from build123d import *

# Parameters (mm, degrees)
SKETCH1_R           = 14
BOSS_EXTRUDE1_DEPTH = 5
BOSS_EXTRUDE3_DEPTH = 20
SKETCH3_R           = 8.5
CUT_EXTRUDE1_DEPTH  = 26
SKETCH5_W           = 4
SKETCH5_H           = 11.5
CUT_EXTRUDE3_DEPTH  = 26
SKETCH6_R           = 1.5
CUT_EXTRUDE4_DEPTH  = 6
CIRPATTERN1_COUNT   = 3
FILLET1_R           = 1.5


with BuildPart() as part:
    # Sketch1 → Boss-Extrude1 (new body)
    with BuildSketch(Plane.XY):
        Circle(SKETCH1_R)
    extrude(amount=BOSS_EXTRUDE1_DEPTH)

    # Sketch2 → Boss-Extrude3 (add)
    with BuildSketch(Plane.XY.offset(5)):
        with BuildLine():
            Line((2.5, -9.16515139), (2.5, -12.16515139))
            Line((2.5, -12.16515139), (-2.5, -12.16515139))
            Line((-2.5, -12.16515139), (-2.5, -9.16515139))
            ThreePointArc((-2.5, -9.16515139), (0, 9.5), (2.5, -9.16515139))
        make_face()
    extrude(amount=BOSS_EXTRUDE3_DEPTH)

    # Sketch3 → Cut-Extrude1 (cut, through all)
    with BuildSketch(Plane.XY.offset(25)):
        Circle(SKETCH3_R)
    extrude(amount=-CUT_EXTRUDE1_DEPTH, mode=Mode.SUBTRACT)

    # Sketch5 → Cut-Extrude3 (cut, through all)
    with BuildSketch(Plane.XY.offset(25)):
        with Locations((0, -5.75)):
            Rectangle(SKETCH5_W, SKETCH5_H)
    extrude(amount=-CUT_EXTRUDE3_DEPTH, mode=Mode.SUBTRACT)

    # Sketch6 → Cut-Extrude4 (cut, through all)
    with BuildSketch(Plane.XY.offset(5)):
        with Locations((0, 11.75)):
            Circle(SKETCH6_R)
    cut_extrude4 = extrude(amount=-CUT_EXTRUDE4_DEPTH, mode=Mode.SUBTRACT)

    # CirPattern1: Cut-Extrude4 ×3 about axis
    cirpattern1_axis = Axis((0, 0, 0), (0, 0, 1))
    for i in range(1, CIRPATTERN1_COUNT):
        add(cut_extrude4.rotate(cirpattern1_axis, i * 360 / CIRPATTERN1_COUNT), mode=Mode.SUBTRACT)

    # Fillet1
    fillet1_edges = [part.edges().sort_by_distance(p)[0] for p in [
        (2, -8.261355821, 12.5),
        (-2, -8.261355821, 12.5),
    ]]
    fillet(fillet1_edges, radius=FILLET1_R)


solid = part.part
The listing builds one solid part. Answer for the finished solid, in the listing's coordinates (mm). A direction names the side the tool comes from. Give positions to 0.01 mm unless a question says otherwise; leave off trailing zeros. Loops run counter-clockwise (first coordinate to the right, second up) from the corner with the lowest first, then second, coordinate; pieces in that order, holes last.
Item 1: Each of these flat-tipped pins is pushed along its axis until it touches: pin 1 Ø1.5 at (x, z) = (-7, 14.5) entering from -Y; pin 2 Ø4.5 at (x, z) = (-0.5, 10.5) entering from +Y; pin 3 Ø12 at (y, z) = (-6, 21.5) entering from -X; pin 4 Ø5 at (y, z) = (0.5, 3.5) entering from +X. Where does it stop, or does it pass through?
Derived:
pin 1: stops at y = -7.15
pin 2: stops at y = 9.5
pin 3: stops at x = -9.5
pin 4: stops at x = 14
Item 2: Find the intervals of material crossed by line 1 along X through (y, z) = (-10.5, 6); line 2 along X through (y, z) = (-6.25, 3); line 3 along X through (y, z) = (0, 13), in increasing order.
Derived:
line 1: x = -2.5 to -2, 2 to 2.5
line 2: x = -12.53 to -11.63, -8.72 to -5.76, 5.76 to 8.72, 11.63 to 12.53
line 3: x = -9.5 to -8.5, 8.5 to 9.5
Item 3: Determine the mould class of faces 1 (the cylindrical face through (-0.382, 9.492, 14.86)), 2 (the flat face through (-2, -10, 13)), 3 (the flat face through (4, -8, 25)) for opening direction Y: +Y half, -Y half, draft (parallel to the pull), parting line (faces both ways), or undercut.
Derived:
face 1: parting line
face 2: undercut
face 3: draft
Item 4: A cutting plane is placed at B-B (y = 0). Give the vertices of the cut face in (x, z), then the cut area to 3 significant figures.
Derived:
outline: (-14, 0) - (-8.5, 0) - (-8.5, 25) - (-9.5, 25) - (-9.5, 5) - (-14, 5) - close; (8.5, 0) - (14, 0) - (14, 5) - (9.5, 5) - (9.5, 25) - (8.5, 25) - close
area: 95.0 mm2
Item 5: A cutting plane is placed at D-D (x = 10.25). Give the vertices of the cut face in (y, z), then the cut area to 3 significant figures.
Derived:
outline: (-9.54, 0) - (-7.37, 0) - (-7.37, 5) - (-9.54, 5) - close; (-4.38, 0) - (9.54, 0) - (9.54, 5) - (-4.38, 5) - close
area: 80.4 mm2
Item 6: A cutting plane is placed at C-C (z = 21.5). Give the vertices of the cut face in (x, y) (1 decimal).
Derived:
outline: (-2.5, -12.2) - (2.5, -12.2) - (2.5, -9.2) arc R9.5 ccw (long way) to (-2.5, -9.2) - close; hole (-3, -8) arc R1.5 cw to (-2, -9.4) - (-2, -11.5) - (2, -11.5) - (2, -9.4) arc R1.5 cw to (3, -8) arc R8.5 ccw (long way) to start
Item 7: A cutting plane is placed at A-A (x = 0). Give the vertices of the cut face in (y, z), then the cut area to 3 significant figures.
Derived:
outline: (-14, 0) - (-11.5, 0) - (-11.5, 25) - (-12.17, 25) - (-12.17, 5) - (-14, 5) - close; (8.5, 0) - (10.25, 0) - (10.25, 5) - (9.5, 5) - (9.5, 25) - (8.5, 25) - close; (13.25, 0) - (14, 0) - (14, 5) - (13.25, 5) - close
area: 58.3 mm2
Item 8: A tool of negligible diameter and unlimited length cuts with its end or side. For faces 4 (the flat face through (-2.5, -11, 15)), 5 (the flat face through (0, -12.165, 15)), 6 (the flat face through (2.5, -11, 15)), 7 (the cylindrical face through (-2.26, -8.52, 12.68)), from which of +Z, -Z, +X, -X, +Y, -Y can it reach the whole face along a straight path? Write none if from no direction.
Derived:
face 4: +Z, -X, -Y
face 5: +Z, +X, -X, -Y
face 6: +Z, +X, -Y
face 7: +Z, -Z
